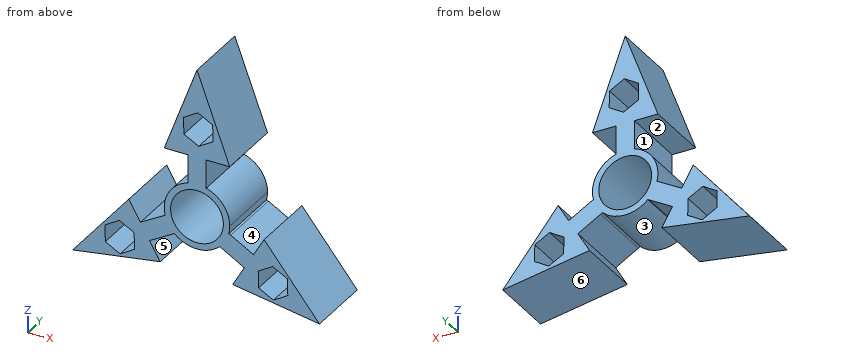
from build123d import *

# Parameters (mm, degrees)
F0_R     = 9.865157
F1_DEPTH = 25


with BuildPart() as f1:
    # F0 (on Front) → F1 (new body)
    with BuildSketch(Plane.XZ):
        with BuildLine():
            ThreePointArc((-3.427112, 11.741537), (0, 12.231467), (3.427112, 11.741537))
            Line((3.427112, 11.741537), (3.427112, 12.56425))
            Line((3.427112, 12.56425), (3.427112, 22.406213))
            Line((3.427112, 22.406213), (12.229432, 22.406213))
            Line((12.229432, 22.406213), (0, 55.397243))
            Line((0, 55.397243), (-12.229432, 22.406213))
            Line((-12.229432, 22.406213), (-3.427112, 22.406213))
            Line((-3.427112, 22.406213), (-3.427112, 12.56425))
            Line((-3.427112, 12.56425), (-3.427112, 11.741537))
        make_face()
        Polygon((5.999969, 30.045177), (0.627875, 26.767383), (-4.896825, 29.780857), (-5.049431, 36.072124), (0.322664, 39.349918), (5.847364, 36.336445), align=None, mode=Mode.SUBTRACT)
        with BuildLine():
            ThreePointArc((-8.454913, -8.838734), (-10.589397, -6.121556), (-11.878826, -2.915866))
            Line((-11.878826, -2.915866), (-12.594515, -3.314159))
            Line((-12.594515, -3.314159), (-21.117905, -8.23514))
            Line((-21.117905, -8.23514), (-25.446913, -0.737079))
            Line((-25.446913, -0.737079), (-46.428616, -26.044891))
            Line((-46.428616, -26.044891), (-13.736432, -21.020227))
            Line((-13.736432, -21.020227), (-17.690794, -14.171072))
            Line((-17.690794, -14.171072), (-9.167404, -9.250091))
            Line((-9.167404, -9.250091), (-8.454913, -8.838734))
        make_face()
        Polygon((-23.342566, -19.131204), (-28.714661, -22.408998), (-34.239361, -19.395524), (-34.391966, -13.104257), (-29.019872, -9.826463), (-23.495171, -12.839936), align=None, mode=Mode.SUBTRACT)
        with BuildLine():
            Line((12.594515, -3.314159), (11.849696, -3.032078))
            ThreePointArc((11.849696, -3.032078), (10.55929, -6.173345), (8.454913, -8.838734))
            Line((8.454913, -8.838734), (9.167404, -9.250091))
            Line((9.167404, -9.250091), (17.690794, -14.171072))
            Line((17.690794, -14.171072), (13.322571, -21.737055))
            Line((13.322571, -21.737055), (45.757505, -27.258412))
            Line((45.757505, -27.258412), (25.072267, -1.385986))
            Line((25.072267, -1.385986), (21.117905, -8.23514))
            Line((21.117905, -8.23514), (12.594515, -3.314159))
        make_face()
        Polygon((28.239391, -10.649653), (33.764091, -13.663127), (33.916697, -19.954394), (28.544602, -23.232188), (23.019902, -20.218715), (22.867297, -13.927447), align=None, mode=Mode.SUBTRACT)
        with BuildLine():
            ThreePointArc((11.849696, -3.032078), (12.135649, -1.528009), (12.231467, 0))
            ThreePointArc((12.231467, 0), (9.785893, 7.337921), (3.427112, 11.741537))
            ThreePointArc((3.427112, 11.741537), (0, 12.231467), (-3.427112, 11.741537))
            ThreePointArc((-3.427112, 11.741537), (-10.596122, 6.109909), (-11.878826, -2.915866))
            ThreePointArc((-11.878826, -2.915866), (-10.589397, -6.121556), (-8.454913, -8.838734))
            ThreePointArc((-8.454913, -8.838734), (0, -12.231467), (8.454913, -8.838734))
            ThreePointArc((8.454913, -8.838734), (10.55929, -6.173345), (11.849696, -3.032078))
        make_face()
        Circle(F0_R, mode=Mode.SUBTRACT)
    extrude(amount=F1_DEPTH)


solid = f1.part
Source: CAD feature listing. Evaluate the final solid. Frame: model axes, mm. Face numbers are marked on the shaded views. A direction names the side the tool comes from. Round coordinates to 2 decimals unless told otherwise and drop trailing zeros. Loops run counter-clockwise (first coordinate to the right, second up) from the corner with the lowest first, then second, coordinate; pieces in that order, holes last. Notation, with made-up numbers: (-20, -13.75) - (22, -13.75) arc R20 ccw to (22, -2.75) - close; hole circle Ø10 at (45.5, -14). An arc over 180 degrees is marked (long way). Write item = value, one per line. Start each with the question number.
(1) Ray query, line 1 along X through (y, z) = (-22, -17); line 2 along X through (y, z) = (-17.75, -4.5); line 3 along Z through (x, y) = (26.5, -19.5). Return the intervals inside material, ascending. Write a range as from..to.
(2) Set-up query: the marked faces 4, 5 and 6. Return all of +Z, -Z, +X, -X, +Y, -Y with unobstructed straight access to the full face (end or side cutting, diameter ignored); none if empty.
(3) Section query A-A, the plane x = 15. Output: boundary loops of the cut face in (y, z), plus the area to 3 significant figures.
(4) Section query B-B, the plane y = -6.5. State how many separate pieces and enclosed holes the cut face has, plus the area to 3 significant figures.
(5) Pin query (flat end, axial travel): pin 1 (3 mm diameter, centred on y = -3, z = 18.5, fed in from +X); pin 2 (1.5 mm diameter, centred on y = -18.5, z = 37, fed in from -X); pin 3 (9.5 mm diameter, centred on x = 9.5, y = -10.5, fed in from -Z); pin 4 (1 mm diameter, centred on x = -11.5, z = 20, fed in from +Y). Return the tip coordinate at first contact, or that it passes through.
(6) Pull-direction query (X, two-part tool) for the marked faces 1, 2 and 3; classes: +X half, -X half, draft (parallel to the pull), parting line (faces both ways), or undercut.
(7) Section query D-D, the plane x = 31.5. Output: boundary loops of the cut face in (y, z), plus the area to 3 significant figures.
(8) Section query C-C, the plane z = -5. Output: boundary loops of the cut face in (x, y).
Conclusion:
q1.line_1 = -38.93..-34.3, -23.39..-16.06, 16.06..22.94, 33.85..37.56
q1.line_2 = -28.57..-23.27, -14.65..-8.78, 8.78..14.65, 23.27..27.56
q1.line_3 = -23.98..-22.12, -11.71..-3.17
q2.face_4 = +Z, +Y, -Y
q2.face_5 = +Y, -Y
q2.face_6 = -Z, +Y, -Y
q3.outline = (-25, -22.02) - (0, -22.02) - (0, -18.83) - (-25, -18.83) - close; (-25, -12.62) - (0, -12.62) - (0, -4.7) - (-25, -4.7) - close
q3.area = 278 mm2
q4.separate_pieces = 1
q4.enclosed_holes = 4
q4.area = 1,190 mm2
q5.pin_1 = 3.43
q5.pin_2 = -7.1
q5.pin_3 = -21.89
q5.pin_4 = through
q6.face_1 = -X half
q6.face_2 = draft
q6.face_3 = undercut
q7.outline = (-25, -24.83) - (0, -24.83) - (0, -21.43) - (-25, -21.43) - close; (-25, -12.43) - (0, -12.43) - (0, -9.43) - (-25, -9.43) - close
q7.area = 160 mm2
q8.outline = (-28.98, -25) - (-22.99, -25) - (-22.99, 0) - (-28.98, 0) - close; (-15.51, -25) - (-8.5, -25) - (-8.5, 0) - (-15.51, 0) - close; (8.5, -25) - (15.51, -25) - (15.51, 0) - (8.5, 0) - close; (22.99, -25) - (27.96, -25) - (27.96, 0) - (22.99, 0) - close
